Verification items for the finished model (mm, model axes). A direction names the side the tool comes from. Give positions to 0.01 mm unless a question says otherwise; leave off trailing zeros. Loops run counter-clockwise (first coordinate to the right, second up) from the corner with the lowest first, then second, coordinate; pieces in that order, holes last. Notation, with made-up numbers: M -37.75,72.5 L -11.75,72.5 A29 ccw -11.75,102.5 Z; hole C 53,-12.75 d8. An arc over 180 degrees is marked long. Answer in a Markdown table with one row per item.
```python
from build123d import *


with BuildPart() as part:
    # 草图3 → 旋转1 (revolve)
    with BuildSketch(Plane(origin=(0, 0, 0), x_dir=(0, 0, -1), z_dir=(1, 0, 0)), mode=Mode.PRIVATE) as revolve_1_sk:
        with BuildLine():
            Line((12.5, 0), (15.5, 0))
            Line((15.5, 0), (15.5, 3.5))
            Line((15.5, 3.5), (14.45, 4))
            Line((14.45, 4), (13.4, 4))
            Line((13.4, 4), (13.4, 3.5))
            Line((13.4, 3.5), (12.5, 3.5))
            Line((12.5, 3.5), (12.5, 4))
            Line((12.5, 4), (0, 4))
            Line((0, 4), (-4.333333333, 4))
            ThreePointArc((-4.333333333, 4), (-4.451184464, 4.048815536), (-4.5, 4.166666667))
            Line((-4.5, 4.166666667), (-4.5, 6.116666667))
            Line((-4.5, 6.116666667), (-4.633333333, 6.25))
            Line((-4.633333333, 6.25), (-6.7, 6.25))
            Line((-6.7, 6.25), (-7, 5.95))
            Line((-7, 5.95), (-7, 0))
            Line((-7, 0), (12.5, 0))
        make_face()
    revolve(revolve_1_sk.sketch.rotate(Axis((0, 0, 7), (0, 0, -1)), 90), axis=Axis((0, 0, 7), (0, 0, -1)))


solid = part.part
```
Item 1: Sectioned sample at A-A (y = 0). Record the cut outline in (x, z), and give its area (3 significant figures).
Reported:
| item | result |
|---|---|
| outline | M -6.25,4.63 L -6.12,4.5 L -4.17,4.5 A0.17 cw -4,4.33 L -4,-12.5 L -3.5,-12.5 L -3.5,-13.4 L -4,-13.4 L -4,-14.45 L -3.5,-15.5 L 3.5,-15.5 L 4,-14.45 L 4,-13.4 L 3.5,-13.4 L 3.5,-12.5 L 4,-12.5 L 4,4.33 A0.17 cw 4.17,4.5 L 6.12,4.5 L 6.25,4.63 L 6.25,6.7 L 5.95,7 L -5.95,7 L -6.25,6.7 Z |
| area | 190 mm^2 |
Item 2: Scan lines: L1, parallel to Z at x = -5.25, y = -0.75; L2, parallel to Y at x = 3, z = -11; L3, parallel to Y at x = 3.5, z = -5.25. Record each from-to range of solid material in increasing order. Write a range as [from, to].
Reported:
| item | result |
|---|---|
| L1 | z = [4.5, 7] |
| L2 | y = [-2.65, 2.65] |
| L3 | y = [-1.94, 1.94] |
Item 3: Tool access check on faces 5 (the flat face through (0, 0, -15.5)), 6 (the cylindrical face through (-0.867, 3.905, -13.918)). Record the directions out of +Z, -Z, +X, -X, +Y, -Y that give a thin tool (end or side, any length) a straight path to the whole face; none if there is none.
Reported:
| item | result |
|---|---|
| face 5 | -Z, +X, -X, +Y, -Y |
| face 6 | -Z |
Item 4: Sectioned sample at C-C (z = 5.5). Record the cut outline in (x, y).
Reported:
| item | result |
|---|---|
| outline | C 0,0 d12.5 |
Item 5: Sectioned sample at D-D (z = -10.5). Record the cut outline in (x, y), and give its area (3 significant figures).
Reported:
| item | result |
|---|---|
| outline | C 0,0 d8 |
| area | 50.3 mm^2 |
Item 6: Release check for a two-part mould opening along Z. For faces 1 (the flat face through (-3, 4, 4.5)), 2 (the cylindrical face through (5.96, -1.88, 5.68)), 3 (the cylindrical face through (1.615, 3.105, -12.944)), 4 (the flat face through (0, 0, 7)) record: released by +Z, released by -Z, zero draft, split by the parting line, or undercut.
Reported:
| item | result |
|---|---|
| face 1 | released by -Z |
| face 2 | zero draft |
| face 3 | undercut |
| face 4 | released by +Z |
